Geometry: final body of the model. Coordinates: model frame, mm. Face numbers are marked on the shaded views. A direction names the side the tool comes from. Round coordinates to 2 decimals unless told otherwise and drop trailing zeros. Order: outer loops, then holes, each group sorted by start corner. A loop starts at its lowest first (then second) coordinate and runs counter-clockwise, first axis right, second up. Notation, with made-up numbers: (68, -8.5) -> (125, -8.5) arc R13 cw to (125, 9.5) -> close; hole circle Ø10 at (27, 62). An arc over 180 degrees is marked (long way). Put each result on its own line as item: value.
```python
from build123d import *

# Parameters (mm, degrees)
SKETCH1_W               = 50.8
SKETCH1_H               = 25.4
BOSS_EXTRUDE1_DEPTH     = 25.4
SHELL1_T                = -1.524
SKETCH2_R               = 0.762
BOSS_EXTRUDE2_DEPTH     = 0.889
SKETCH3_W               = 15.24
SKETCH3_H               = 13.97
CUT_EXTRUDE1_DEPTH      = 23.876
SKETCH4_R               = 7.62
CUT_EXTRUDE2_DEPTH      = 23.876
CUT_EXTRUDE3_DEPTH      = 39.698340029
CUT_EXTRUDE3_DEPTH_BACK = 39.698340029
SKETCH5_R               = 8.73125


with BuildPart() as part:
    # Sketch1 → Boss-Extrude1 (new body)
    with BuildSketch(Plane.XY):
        Rectangle(SKETCH1_W, SKETCH1_H)
    extrude(amount=BOSS_EXTRUDE1_DEPTH)

    # Shell1
    shell1_openings = [part.faces().sort_by_distance(p)[0] for p in [
        (0, 0, 0),
    ]]
    offset(amount=SHELL1_T, openings=shell1_openings, kind=Kind.INTERSECTION)

    # Sketch2 → Boss-Extrude2 (add)
    with BuildSketch(Plane(origin=(0, 0, 0), x_dir=(-1, 0, 0), z_dir=(0, 0, -1))):
        with Locations(Location((-24.511, 11.811, 0), (0, 0, 180))):
            Circle(SKETCH2_R)
        with Locations(Location((24.511, 11.811, 0), (0, 0, 180))):
            Circle(SKETCH2_R)
        with Locations(Location((24.511, -11.811, 0), (0, 0, 180))):
            Circle(SKETCH2_R)
        with Locations(Location((-24.511, -11.811, 0), (0, 0, 180))):
            Circle(SKETCH2_R)
    extrude(amount=BOSS_EXTRUDE2_DEPTH)

    # Sketch3 → Cut-Extrude1 (cut)
    with BuildSketch(Plane(origin=(0, -12.7, 0), x_dir=(-1, 0, 0), z_dir=(0, -1, 0))):
        with Locations((0, -6.985)):
            Rectangle(SKETCH3_W, SKETCH3_H)
    extrude(amount=-CUT_EXTRUDE1_DEPTH, mode=Mode.SUBTRACT)

    # Sketch4 → Cut-Extrude2 (cut)
    with BuildSketch(Plane(origin=(0, 12.7, 0), x_dir=(1, 0, 0), z_dir=(0, 1, 0))):
        with Locations(Location((0, -12.7, 0), (0, 0, 270))):
            Circle(SKETCH4_R)
    extrude(amount=-CUT_EXTRUDE2_DEPTH, mode=Mode.SUBTRACT)

    # Sketch5 → Cut-Extrude3 (cut, two sides: drawn at the far end of the back side and taken through both)
    with BuildSketch(Plane.XY.offset(25.4).offset(-CUT_EXTRUDE3_DEPTH_BACK)):
        with Locations((-13.43025, -1.42875)):
            Circle(SKETCH5_R)
        with Locations((13.43025, -1.42875)):
            Circle(SKETCH5_R)
    extrude(amount=CUT_EXTRUDE3_DEPTH + CUT_EXTRUDE3_DEPTH_BACK, mode=Mode.SUBTRACT)


solid = part.part
```
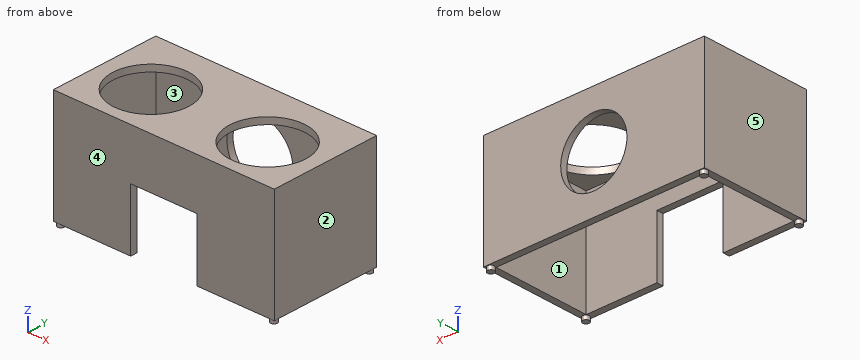
1. Cut plane A-A on z = 12.7. Return loops of the section in (x, y).
Ans:
outline: (-25.4, -12.7) -> (-7.62, -12.7) -> (-7.62, -11.18) -> (-23.88, -11.18) -> (-23.88, 11.18) -> (-7.62, 11.18) -> (-7.62, 12.7) -> (-25.4, 12.7) -> close; (7.62, -12.7) -> (25.4, -12.7) -> (25.4, 12.7) -> (7.62, 12.7) -> (7.62, 11.18) -> (23.88, 11.18) -> (23.88, -11.18) -> (7.62, -11.18) -> close
2. Cut plane C-C on y = -7. Return loops of the section in (x, z).
Ans:
outline: (-25.4, 0) -> (-23.88, 0) -> (-23.88, 23.88) -> (-20.15, 23.88) -> (-20.15, 25.4) -> (-25.4, 25.4) -> close; (-6.71, 23.88) -> (6.71, 23.88) -> (6.71, 25.4) -> (-6.71, 25.4) -> close; (20.15, 23.88) -> (23.88, 23.88) -> (23.88, 0) -> (25.4, 0) -> (25.4, 25.4) -> (20.15, 25.4) -> close
3. Set-up query: the marked faces 1 and 2. Return all of +Z, -Z, +X, -X, +Y, -Y with unobstructed straight access to the full face (end or side cutting, diameter ignored); none if empty.
Ans:
face 1: -Z
face 2: +Z, -Z, +X, +Y, -Y
4. Material intervals for probe 1 along Y at (x, z) = (-12, 0.5); probe 2 along X at (y, z) = (-0.75, 18.25); probe 3 along X at (y, z) = (11.95, 12.7), sorted ascending.
Ans:
probe 1: -12.7 to -11.18, 11.18 to 12.7
probe 2: -25.4 to -23.88, 23.88 to 25.4
probe 3: -25.4 to -7.62, 7.62 to 25.4
5. Cut plane D-D on y = 9.25. Return loops of the section in (x, z).
Ans:
outline: (-25.4, 0) -> (-23.88, 0) -> (-23.88, 23.88) -> (23.88, 23.88) -> (23.88, 0) -> (25.4, 0) -> (25.4, 25.4) -> (-25.4, 25.4) -> close
6. Cut plane B-B on x = 14. Return loops of the section in (y, z), and give its area (3 significant figures).
Ans:
outline: (-12.7, 0) -> (-11.18, 0) -> (-11.18, 23.88) -> (-10.14, 23.88) -> (-10.14, 25.4) -> (-12.7, 25.4) -> close; (7.28, 23.88) -> (11.18, 23.88) -> (11.18, 0) -> (12.7, 0) -> (12.7, 25.4) -> (7.28, 25.4) -> close
area: 84.9 mm²
7. Contact query for flat-ended pins moving along their axis: P1, Ø2, axis at x = -17, y = 8.5, coming from the -Z side; P2, Ø14, axis at x = 13.43, y = -1.43, coming from the +Z side; P3, Ø9, axis at x = 0, z = 12.7, coming from the +Y side; P4, Ø0.5, axis at x = 1, y = -12.5, coming from the -Z side. Output: stop coordinate, or through.
Ans:
P1: z = 23.88
P2: through
P3: y = -11.18
P4: z = 13.97
8. Draft query along X for the marked faces 3, 4 and 5. Return one class per face: +X half, -X half, draft (parallel to the pull), parting line (faces both ways), or undercut.
Ans:
face 3: undercut
face 4: draft
face 5: -X half
